```python
from build123d import *

# Parameters (mm, degrees)
BASE_FLANGE1_DEPTH           = 3.175
M6_CLEARANCE_HOLE1_D         = 6.6
EDGE_FLANGE1_DEPTH           = 16.378
EDGE_FLANGE2_STRIP_W         = 14.1732
EDGE_FLANGE2_STRIP_H         = 3.175
EDGE_FLANGE2_STRIP_CUT_DEPTH = 16.378
EDGE_FLANGE2_DEPTH           = 16.378
M5_CLEARANCE_HOLE1_D         = 5.5
FILLET1_R                    = 2.54
FILLET2_R                    = 6.35


# Sheet-metal steps are written as plain solids
with BuildPart() as part:
    # Sketch1 → Base-Flange1 (new body)
    with BuildSketch(Plane.XY):
        Polygon((52.8905, -45.562600001), (36.5125, -45.562600001), (36.5125, -29.184600001), (61.9125, -29.184600001), (61.9125, -45.562600001), align=None)
    extrude(amount=-BASE_FLANGE1_DEPTH)

    # M6 Clearance Hole1 (through all)
    with Locations(Plane.XY):
        with Locations((46.0375, -37.373600001)):
            Hole(M6_CLEARANCE_HOLE1_D / 2)

    # Edge-Flange1 section (across the edge) → Edge-Flange1 (add)
    with BuildSketch(Plane(origin=(62.6491, -45.562600001, 0), x_dir=(-1, 0, 0), z_dir=(0, 1, 0))):
        with BuildLine():
            Line((-3.175, 0.7366), (-3.175, 32.0779))
            Line((-3.175, 32.0779), (0, 32.0779))
            Line((0, 32.0779), (0, 0.7366))
            ThreePointArc((0, 0.7366), (0.215745145, 0.215745145), (0.7366, 0))
            Line((0.7366, 0), (0.7366, -3.175))
            ThreePointArc((0.7366, -3.175), (-2.029318885, -2.029318885), (-3.175, 0.7366))
        make_face()
    extrude(amount=EDGE_FLANGE1_DEPTH)

    # Edge-Flange2 strip (across the edge) → Edge-Flange2 strip cut (cut)
    with BuildSketch(Plane(origin=(65.8241, -29.184600001, 32.0779), x_dir=(0, 0, -1), z_dir=(0, -1, 0))):
        with Locations((-6.35, -1.5875)):
            Rectangle(EDGE_FLANGE2_STRIP_W, EDGE_FLANGE2_STRIP_H)
    extrude(amount=EDGE_FLANGE2_STRIP_CUT_DEPTH, mode=Mode.SUBTRACT)

    # Edge-Flange2 section (across the edge) → Edge-Flange2 (add)
    with BuildSketch(Plane(origin=(65.8241, -29.184600001, 32.0779), x_dir=(0, 0, -1), z_dir=(0, -1, 0))):
        with BuildLine():
            Line((-3.175, 0.7366), (-3.175, 34.925))
            Line((-3.175, 34.925), (0, 34.925))
            Line((0, 34.925), (0, 0.7366))
            ThreePointArc((0, 0.7366), (0.215745145, 0.215745145), (0.7366, 0))
            Line((0.7366, 0), (0.7366, -3.175))
            ThreePointArc((0.7366, -3.175), (-2.029318885, -2.029318885), (-3.175, 0.7366))
        make_face()
    extrude(amount=EDGE_FLANGE2_DEPTH)

    # M5 Clearance Hole1 (through all)
    with Locations(Plane.XY.offset(35.2529)):
        with Locations((94.5499, -37.373600001)):
            Hole(M5_CLEARANCE_HOLE1_D / 2)

    # Fillet1
    fillet1_edges = [part.edges().sort_by_distance(p)[0] for p in [
        (100.7491, -29.184600001, 33.6654),
        (36.5125, -45.562600001, -1.5875),
        (36.5125, -29.184600001, -1.5875),
    ]]
    fillet(fillet1_edges, radius=FILLET1_R)

    # Fillet2
    fillet2_edges = [part.edges().sort_by_distance(p)[0] for p in [
        (100.7491, -45.562600001, 33.6654),
    ]]
    fillet(fillet2_edges, radius=FILLET2_R)


solid = part.part
```
The model under review builds one solid part; all positions refer to its coordinate system, in mm. A direction names the side the tool comes from. Give positions to 0.01 mm unless a question says otherwise; leave off trailing zeros. Order: outer loops, then holes, each group sorted by start corner. A loop starts at its lowest first (then second) coordinate and runs counter-clockwise, first axis right, second up. Notation, with made-up numbers: (40, 84.5) - (51, 84.5) arc R31 ccw to (51, 116.5) - close; hole circle Ø9 at (-31, 19.25). An arc over 180 degrees is marked (long way). Use CSV: the item, a comma, the result in double quotes. Start each with the question number.
Q1. We need section A-A, the plane y = -38. Write out the cut boundary in (x, z) (1 decimal), and give its area (3 significant figures).
Q2. Tool access review of faces 4 (the flat face through (65.824, -37, 16)), 5 (the flat face through (49, -35, 0)), 6 (the cylindrical face through (37.276, -29.909, -1.61)): name each direction out of +Z, -Z, +X, -X, +Y, -Y from which nothing blocks a thin tool from reaching the whole face with its end or side.
Q3. We need section D-D, the plane x = 81. Write out the cut boundary in (y, z), and give its area (3 significant figures).
Q4. We need section C-C, the plane y = -32.75. Write out the cut boundary in (x, z) (1 decimal).
Q5. Clearance check with flat-ended pins moving along their axes: pin 1 Ø7 at (x, y) = (94.55, -37.37) entering from +Z; pin 2 Ø8 at (y, z) = (-38.5, 8.5) entering from +X; pin 3 Ø8 at (x, y) = (60, -34) entering from +Z; pin 4 Ø4 at (x, y) = (46.04, -37.37) entering from -Z. State where each tip first meets the part, or that it passes through.
Q6. The part is to be moulded in two halves that separate along Y. For faces 1 (the cylindrical face through (49.334, -37.229, -1.61)), 2 (the cylindrical face through (37.28, -44.84, -1.61)), 3 (the flat face through (84, -37, 32.078)), say which applies: +Y half, -Y half, draft (parallel to the pull), parting line (faces both ways), or undercut.
Q7. We need section B-B, the plane x = 44. Write out the cut boundary in (y, z) (3 decimals).
Q8. To check wall thickness, follow line 1 along Z through (x, y) = (73, -34.75); line 2 along X through (y, z) = (-39.5, 22); line 3 along Z through (x, y) = (57, -33.5) (3 decimals). State the ranges of each line that lie inside material, in increasing order. Write a range as [from, to].
Outcome:
1,outline,"(36.5, -3.2) - (42.8, -3.2) - (42.8, 0) - (36.5, 0) - close; (49.3, -3.2) - (61.9, -3.2) arc R3.9 ccw to (65.8, 0.7) - (65.8, 31.3) arc R0.7 cw to (66.6, 32.1) - (91.9, 32.1) - (91.9, 35.3) - (66.6, 35.3) arc R3.9 ccw to (62.6, 31.3) - (62.6, 0.7) arc R0.7 cw to (61.9, 0) - (49.3, 0) - close; (97.2, 32.1) - (100.7, 32.1) - (100.7, 35.3) - (97.2, 35.3) - close"
1,area,"272 mm^2"
2,face 4,"-Z, +X, +Y, -Y"
2,face 5,"+Z, -X, +Y, -Y"
2,face 6,"+Z, -Z, -X, +Y"
3,outline,"(-45.56, 32.08) - (-29.18, 32.08) - (-29.18, 35.25) - (-45.56, 35.25) - close"
3,area,"52.0 mm^2"
4,outline,"(36.5, -3.2) - (61.9, -3.2) arc R3.9 ccw to (65.8, 0.7) - (65.8, 31.3) arc R0.7 cw to (66.6, 32.1) - (100.7, 32.1) - (100.7, 35.3) - (66.6, 35.3) arc R3.9 ccw to (62.6, 31.3) - (62.6, 0.7) arc R0.7 cw to (61.9, 0) - (36.5, 0) - close"
5,pin 1,"stops at z = 35.25"
5,pin 2,"stops at x = 65.82"
5,pin 3,"stops at z = 34.3"
5,pin 4,"passes through"
6,face 1,"undercut"
6,face 2,"-Y half"
6,face 3,"draft"
7,outline,"(-45.563, -3.175) - (-39.969, -3.175) - (-39.969, 0) - (-45.563, 0) - close; (-34.778, -3.175) - (-29.185, -3.175) - (-29.185, 0) - (-34.778, 0) - close"
8,line 1,"z = [32.08, 35.25]"
8,line 2,"x = [62.65, 65.82]"
8,line 3,"z = [-3.175, 0]"
